```python
from build123d import *

# Parameters (mm, degrees)
SKETCH2_W           = 5
SKETCH2_H           = 5
BOSS_EXTRUDE1_DEPTH = 5
CUT_EXTRUDE1_DEPTH  = 2.5


with BuildPart() as part:
    # Sketch2 → Boss-Extrude1 (new body)
    with BuildSketch(Plane(origin=(0, 0, 0), x_dir=(1, 0, 0), z_dir=(0, 1, 0))):
        with BuildLine():
            Line((5, 0), (45, 0))
            ThreePointArc((45, 0), (48.535533906, -1.464466094), (50, -5))
            Line((50, -5), (50, -58.6))
            ThreePointArc((50, -58.6), (48.535533906, -62.135533906), (45, -63.6))
            Line((45, -63.6), (5, -63.6))
            ThreePointArc((5, -63.6), (1.464466094, -62.135533906), (0, -58.6))
            Line((0, -58.6), (0, -5))
            ThreePointArc((0, -5), (1.464466094, -1.464466094), (5, 0))
        make_face()
        with Locations((6.5, -56.1)):
            Rectangle(SKETCH2_W, SKETCH2_H, mode=Mode.SUBTRACT)
        with Locations((6.5, -7.5)):
            Rectangle(SKETCH2_W, SKETCH2_H, mode=Mode.SUBTRACT)
    extrude(amount=BOSS_EXTRUDE1_DEPTH)

    # Sketch4 → Cut-Extrude1 (cut)
    with BuildSketch(Plane(origin=(0, 5, 0), x_dir=(1, 0, 0), z_dir=(0, 1, 0))):
        with BuildLine():
            Line((18.377964167, -27.579927161), (7.298442774, -29.636968644))
            ThreePointArc((7.298442774, -29.636968644), (6.008366652, -30.393500731), (5.500039, -31.8))
            ThreePointArc((5.500039, -31.8), (6.008366652, -33.206499269), (7.298442774, -33.963031356))
            Line((7.298442774, -33.963031356), (18.377964167, -36.020072839))
            ThreePointArc((18.377964167, -36.020072839), (19.95165505, -36.84834495), (20.779927161, -38.422035833))
            Line((20.779927161, -38.422035833), (22.836968644, -49.501557226))
            ThreePointArc((22.836968644, -49.501557226), (25, -51.299961), (27.163031356, -49.501557226))
            Line((27.163031356, -49.501557226), (29.220072839, -38.422035833))
            ThreePointArc((29.220072839, -38.422035833), (30.04834495, -36.84834495), (31.622035833, -36.020072839))
            Line((31.622035833, -36.020072839), (42.701557226, -33.963031356))
            ThreePointArc((42.701557226, -33.963031356), (44.499961, -31.8), (42.701557226, -29.636968644))
            Line((42.701557226, -29.636968644), (31.622035833, -27.579927161))
            ThreePointArc((31.622035833, -27.579927161), (30.04834495, -26.75165505), (29.220072839, -25.177964167))
            Line((29.220072839, -25.177964167), (27.163031356, -14.098442774))
            ThreePointArc((27.163031356, -14.098442774), (25, -12.300039), (22.836968644, -14.098442774))
            Line((22.836968644, -14.098442774), (20.779927161, -25.177964167))
            ThreePointArc((20.779927161, -25.177964167), (19.95165505, -26.75165505), (18.377964167, -27.579927161))
        make_face()
    extrude(amount=-CUT_EXTRUDE1_DEPTH, mode=Mode.SUBTRACT)


solid = part.part
```
Geometry: final body of the model. Coordinates: model frame, mm. A direction names the side the tool comes from. Round coordinates to 2 decimals unless told otherwise and drop trailing zeros. Order: outer loops, then holes, each group sorted by start corner. A loop starts at its lowest first (then second) coordinate and runs counter-clockwise, first axis right, second up. Notation, with made-up numbers: M 28,60.5 L 87,60.5 A15 cw 87,67.5 Z; hole C 89.5,14.25 d3. An arc over 180 degrees is marked long. Use one line per item in the form item = value. Start each with the question number.
Q1. Mould query, pull axis X, two halves, no side actions, for faces 1 (the face through (48.57, 2.46, 62.1)), 2 (the face through (12.761, 3.768, 34.977)), 3 (the face through (25, 0, 31)), 4 (the face through (12.916, 3.768, 28.594)). Classes: +X half, -X half, draft (parallel to the pull), parting line (faces both ways), or undercut.
Q2. Cut plane D-D (x = 14). Return loops of the section in (y, z).
Q3. Material intervals for line 1 (Z direction, x = 6.5, y = 0.9); line 2 (X direction, y = 1.05, z = 8); line 3 (Y direction, x = 30.5, z = 30), sorted ascending. Write a range as [from, to].
Q4. Access query for faces 5 (the face through (19.9, 3.8, 36.8)), 6 (the face through (6, 2, 58.6)), 7 (the face through (1, 2, 2)). Directions: +Z, -Z, +X, -X, +Y, -Y. A direction counts if a zero-diameter tool reaches every point of the face in a straight line with its end or side. Return the directions, or none.
Q5. Cut plane A-A (z = 9). Return loops of the section in (x, y).
Q6. Cut plane B-B (x = 8). Return loops of the section in (y, z).
Q7. Cut plane C-C (y = 3.75). Count the separate pieces of the cut face and the enclosed holes in it, and give its area (3 significant figures).
Q8. Pin query (flat end, axial travel): pin 1 Ø4 at (x, z) = (19, 31) entering from +Y. Return the tip coordinate at first contact, or that it passes through.
Geometry results:
q1.face_1 = +X half
q1.face_2 = undercut
q1.face_3 = draft
q1.face_4 = undercut
q2.outline = M 0,0 L 5,0 L 5,28.39 L 2.5,28.39 L 2.5,35.21 L 5,35.21 L 5,63.6 L 0,63.6 Z
q3.line_1 = [0, 5], [10, 53.6], [58.6, 63.6]
q3.line_2 = [0, 4], [9, 50]
q3.line_3 = [0, 2.5]
q4.face_5 = +Y
q4.face_6 = +Y, -Y
q4.face_7 = -Z, -X, +Y, -Y
q5.outline = M 0,0 L 4,0 L 4,5 L 0,5 Z; M 9,0 L 50,0 L 50,5 L 9,5 Z
q6.outline = M 0,0 L 5,0 L 5,5 L 0,5 Z; M 0,10 L 5,10 L 5,29.51 L 2.5,29.51 L 2.5,34.09 L 5,34.09 L 5,53.6 L 0,53.6 Z; M 0,58.6 L 5,58.6 L 5,63.6 L 0,63.6 Z
q7.separate_pieces = 1
q7.enclosed_holes = 3
q7.area = 2,640 mm^2
q8.pin_1 = 2.5
